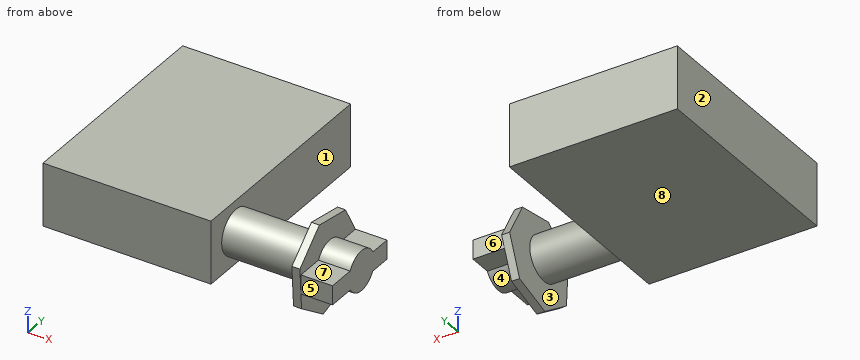
```python
from build123d import *

# Parameters (mm, degrees)
F0_W     = 53.3547988161
F0_H     = 19.9866779149
F1_DEPTH = 69.088
F2_R     = 7.0602732338
F3_DEPTH = 25.4
F5_DEPTH = 2.54
F7_DEPTH = 10.033


with BuildPart() as f1:
    # F0 (on Front) → F1 (new body)
    with BuildSketch(Plane.XZ):
        with Locations((-13.8097074814, 18.6486560851)):
            Rectangle(F0_W, F0_H)
    extrude(amount=F1_DEPTH)

    # F2 (on face) → F3 (join)
    with BuildSketch(Plane.YZ.offset(12.8676919267)):
        with Locations((-56.7260272801, 18.7238119543)):
            Circle(F2_R)
    extrude(amount=F3_DEPTH)

    # F4 (on face) → F5 (join)
    with BuildSketch(Plane.YZ.offset(38.2676919267)):
        Polygon((-46.0683374544, 29.5102504033), (-58.9465306262, 31.6174495083), (-68.6234273353, 22.8626898016), (-67.812126987, 9.838483907), (-57.123555291, 2.3523245085), (-44.6064247416, 6.041442323), (-39.6863899454, 18.1278563919), align=None)
    extrude(amount=F5_DEPTH)

    # F6 (on face) → F7 (join)
    with BuildSketch(Plane.YZ.offset(40.8076919267)):
        with BuildLine():
            ThreePointArc((-59.2542665191, 14.6833357248), (-53.7665337324, 11.5151886184), (-48.2788009457, 14.6833357248))
            Line((-48.2788009457, 14.6833357248), (-59.2542665191, 14.6833357248))
        make_face()
        with BuildLine():
            ThreePointArc((-48.1241693804, 20.7364859485), (-47.6057251813, 19.3354981023), (-47.4296488155, 17.8520735353))
            ThreePointArc((-47.4296488155, 17.8520735353), (-47.6456170701, 16.211802319), (-48.2788009457, 14.6833357248))
            Line((-48.2788009457, 14.6833357248), (-41.1490116824, 14.6833357248))
            Line((-41.1490116824, 14.6833357248), (-41.1490116824, 20.7364859485))
            Line((-41.1490116824, 20.7364859485), (-48.1241693804, 20.7364859485))
        make_face()
        with BuildLine():
            ThreePointArc((-59.2542665191, 14.6833357248), (-60.1013520003, 17.690246581), (-59.4088980844, 20.7364859485))
            Line((-59.4088980844, 20.7364859485), (-68.1139211999, 20.7364859485))
            Line((-68.1139211999, 20.7364859485), (-68.1139211999, 14.6833357248))
            Line((-68.1139211999, 14.6833357248), (-59.2542665191, 14.6833357248))
        make_face()
        with BuildLine():
            Line((-59.4088980844, 20.7364859485), (-48.1241693804, 20.7364859485))
            ThreePointArc((-48.1241693804, 20.7364859485), (-53.7665337324, 24.1889584522), (-59.4088980844, 20.7364859485))
        make_face()
        with BuildLine():
            ThreePointArc((-48.2788009457, 14.6833357248), (-47.6456170701, 16.211802319), (-47.4296488155, 17.8520735353))
            ThreePointArc((-47.4296488155, 17.8520735353), (-47.6057251813, 19.3354981023), (-48.1241693804, 20.7364859485))
            Line((-48.1241693804, 20.7364859485), (-59.4088980844, 20.7364859485))
            ThreePointArc((-59.4088980844, 20.7364859485), (-60.1013520003, 17.690246581), (-59.2542665191, 14.6833357248))
            Line((-59.2542665191, 14.6833357248), (-48.2788009457, 14.6833357248))
        make_face()
    extrude(amount=F7_DEPTH)


solid = f1.part
```
Could you check a few things on this model? Use its own coordinates, in mm. Face numbers are marked on the shaded views. A direction names the side the tool comes from. Round coordinates to 2 decimals unless told otherwise and drop trailing zeros. Loops run counter-clockwise (first coordinate to the right, second up) from the corner with the lowest first, then second, coordinate; pieces in that order, holes last. Notation, with made-up numbers: (89, -26.75) -> (97, -26.75) arc R15 ccw to (97, -4.75) -> close; hole circle Ø9 at (36, -1.75). An arc over 180 degrees is marked (long way). Put each result on its own line as item: value.
Q1. I want a section at C-C on x = -32. Write out the boundary of the cut face in (y, z), and give its area (3 significant figures).
Checks:
outline: (-69.09, 8.66) -> (0, 8.66) -> (0, 28.64) -> (-69.09, 28.64) -> close
area: 1,380 mm2
Q2. Which directions (+Z, -Z, +X, -X, +Y, -Y) give clear straight access to the entire face, cutting with the end or side of a thin tool? Please do the marked faces 5, 6, 7 and 8.
Checks:
face 5: +Z, -Z, +X, -Y
face 6: +Z, -Z, +X, +Y
face 7: +Z, +X, -Y
face 8: -Z, -X, +Y, -Y
Q3. Please list where these lines run through material, in increasing order: line 1 (X direction, y = -30, z = 12.5); line 2 (Z direction, x = -17, y = -17); line 3 (Z direction, x = 45.5, y = -64). Write a range as from..to.
Checks:
line 1: -40.49..12.87
line 2: 8.66..28.64
line 3: 14.68..20.74
Q4. Thinking about a two-plate mould opening in X: for the marked faces 1, 2, 3 and 4, which applies, pulls with the +X half, pulls with the -X half, needs draft (parallel to the pull), parting line crosses it, or undercut?
Checks:
face 1: undercut
face 2: pulls with the -X half
face 3: undercut
face 4: needs draft
Q5. I want a section at B-B on z = 16.25. Write out the boundary of the cut face in (x, y), and give its area (3 significant figures).
Checks:
outline: (-40.49, -69.09) -> (12.87, -69.09) -> (12.87, -63.34) -> (38.27, -63.34) -> (38.27, -68.21) -> (40.81, -68.21) -> (40.81, -68.11) -> (50.84, -68.11) -> (50.84, -41.15) -> (40.81, -41.15) -> (40.81, -40.45) -> (38.27, -40.45) -> (38.27, -50.11) -> (12.87, -50.11) -> (12.87, 0) -> (-40.49, 0) -> close
area: 4,360 mm2
Q6. For pin 1 Ø2 at (x, z) = (-21.5, 15.5) entering from +Y; pin 2 Ø16 at (y, z) = (-31.5, 15.5) entering from +X; pin 3 Ø1.5 at (x, y) = (-17.5, -21.5) entering from -Z; pin 4 Ø5.5 at (x, y) = (47.5, -44) entering from +Z, each with a flat end and sliding along its axis, tell me the tip position at first contact or that it passes through.
Checks:
pin 1: y = 0
pin 2: x = 12.87
pin 3: z = 8.66
pin 4: z = 20.74
Q7. I want a section at D-D on y = -9. Write out the boundary of the cut face in (x, z), and give its area (3 significant figures).
Checks:
outline: (-40.49, 8.66) -> (12.87, 8.66) -> (12.87, 28.64) -> (-40.49, 28.64) -> close
area: 1,070 mm2
Q8. I want a section at A-A on y = -54.5. Write out the boundary of the cut face in (x, z), and give its area (3 significant figures).
Checks:
outline: (-40.49, 8.66) -> (12.87, 8.66) -> (12.87, 12.02) -> (38.27, 12.02) -> (38.27, 3.13) -> (40.81, 3.13) -> (40.81, 11.56) -> (50.84, 11.56) -> (50.84, 24.15) -> (40.81, 24.15) -> (40.81, 30.89) -> (38.27, 30.89) -> (38.27, 25.42) -> (12.87, 25.42) -> (12.87, 28.64) -> (-40.49, 28.64) -> close
area: 1,600 mm2
